Input: part model. Units: mm. Frame: model coordinates. A direction names the side the tool comes from. Round coordinates to 2 decimals unless told otherwise and drop trailing zeros.
Item 1: Mould query, pull axis X, two halves, no side actions, for faces 1 (the flat face through (-12, 50, 13)), 2 (the flat face through (-9, 49, -12.5)), 3 (the cylindrical face through (-14, 18, -13)). Classes: released by +X, released by -X, zero draft, split by the parting line, or undercut.
Item 2: Reachability of faces 4 (the flat face through (6.25, 31, -14)), 5 (the flat face through (14, 31, -6.25)), 6 (the cylindrical face through (-13.732, 49.248, -6.963)) from +Z, -Z, +X, -X, +Y, -Y: full face, straight path, thin tool, end or side. Return the list, or none.
Item 3: Line query: L1, parallel to Y at x = 13.5, z = 8.5; L2, parallel to Z at x = -3.5, y = 47; L3, parallel to Z at x = 3.5, y = 29. Output: solid intervals per line, ascending.
Item 4: First-contact query: pin 1 (2 mm diameter, centred on x = 12, y = 38.5, fed in from +Z); pin 2 (3 mm diameter, centred on y = 44.5, z = 13, fed in from +X); pin 3 (4 mm diameter, centred on x = -4, z = 0, fed in from +Y). Flat tips, straight axial feed; report the tip coordinate or a pass-through.
```python
from build123d import *

# Parameters (mm, degrees)
SKETCH2_W           = 30
SKETCH2_H           = 30
BOSS_EXTRUDE1_DEPTH = 50
SKETCH3_W           = 25
SKETCH3_H           = 25
CUT_EXTRUDE1_DEPTH  = 2.5
FILLET1_R           = 5
SKETCH9_W           = 12.5
SKETCH9_H           = 20.172460503
CUT_EXTRUDE2_DEPTH  = 2.5
CIRPATTERN1_COUNT   = 4
SKETCH10_R          = 21.055389581
CUT_EXTRUDE4_DEPTH  = 5
FILLET2_R           = 2.5


with BuildPart() as part:
    # Sketch2 → Boss-Extrude1 (new body)
    with BuildSketch(Plane(origin=(0, 0, 0), x_dir=(1, 0, 0), z_dir=(0, 1, 0))):
        Rectangle(SKETCH2_W, SKETCH2_H)
    extrude(amount=BOSS_EXTRUDE1_DEPTH)

    # Sketch3 → Cut-Extrude1 (cut)
    with BuildSketch(Plane(origin=(0, 50, 0), x_dir=(1, 0, 0), z_dir=(0, 1, 0))):
        Rectangle(SKETCH3_W, SKETCH3_H)
    extrude(amount=-CUT_EXTRUDE1_DEPTH, mode=Mode.SUBTRACT)

    # Fillet1
    fillet1_edges = [part.edges().sort_by_distance(p)[0] for p in [
        (15, 25, 15),
        (-15, 25, 15),
        (-15, 25, -15),
        (15, 25, -15),
    ]]
    fillet(fillet1_edges, radius=FILLET1_R)

    # Cut-Loft2: read off the stored shape, not the designer's step
    # Cut-Loft2: loft between two sections, ruled curve by curve
    cut_loft2_from = [
        Edge.make_bspline([(0, 0, -12.5), (-25, 0, -12.5), (-25, 0, 12.5), (0, 0, 12.5), (25, 0, 12.5), (25, 0, -12.5), (0, 0, -12.5)], [0, 0, 0, 0, 0.5, 0.5, 0.5, 1, 1, 1, 1], 3, [1, 0.333333333, 0.333333333, 1, 0.333333333, 0.333333333, 1]),
    ]
    cut_loft2_to = [
        Edge.make_bspline([(0.784484005, 47.5, -2.373728048), (-3.962972092, 47.5, -3.942696057), (-5.531940101, 47.5, 0.804760039), (-0.784484005, 47.5, 2.373728048), (3.962972092, 47.5, 3.942696057), (5.531940101, 47.5, -0.804760039), (0.784484005, 47.5, -2.373728048)], [0, 0, 0, 0, 0.5, 0.5, 0.5, 1, 1, 1, 1], 3, [1, 0.333333333, 0.333333333, 1, 0.333333333, 0.333333333, 1]),
    ]
    cut_loft2 = Solid(Shell([*[Face.make_surface_from_curves(cut_loft2_from[k], cut_loft2_to[k]) for k in range(1)], Face(Wire(cut_loft2_from)), Face(Wire(cut_loft2_to))]))
    add(cut_loft2, mode=Mode.SUBTRACT)

    # Sketch9 → Cut-Extrude2 (cut)
    with BuildSketch(Plane.XY.offset(15)):
        with Locations((0, 39.913769749)):
            Rectangle(SKETCH9_W, SKETCH9_H)
    cut_extrude2 = extrude(amount=-CUT_EXTRUDE2_DEPTH, mode=Mode.SUBTRACT)

    # CirPattern1: Cut-Loft2, Cut-Extrude2 ×4 about axis
    cirpattern1_axis = Axis((0, 0, 0), (0, 1, 0))
    add([cut_loft2.rotate(cirpattern1_axis, i * 360 / CIRPATTERN1_COUNT) for i in range(1, CIRPATTERN1_COUNT)], mode=Mode.SUBTRACT)
    add([cut_extrude2.rotate(cirpattern1_axis, i * 360 / CIRPATTERN1_COUNT) for i in range(1, CIRPATTERN1_COUNT)], mode=Mode.SUBTRACT)

    # Sketch10 → Cut-Extrude4 (cut)
    with BuildSketch(Plane(origin=(0, 35, 0), x_dir=(1, 0, 0), z_dir=(0, 1, 0))):
        Circle(SKETCH10_R)
        with BuildLine():
            ThreePointArc((12.5, 10), (11.767766953, 11.767766953), (10, 12.5))
            Line((10, 12.5), (6.25, 12.5))
            Line((6.25, 12.5), (-6.25, 12.5))
            Line((-6.25, 12.5), (-10, 12.5))
            ThreePointArc((-10, 12.5), (-11.767766953, 11.767766953), (-12.5, 10))
            Line((-12.5, 10), (-12.5, 6.25))
            Line((-12.5, 6.25), (-12.5, -6.25))
            Line((-12.5, -6.25), (-12.5, -10))
            ThreePointArc((-12.5, -10), (-11.767766953, -11.767766953), (-10, -12.5))
            Line((-10, -12.5), (-6.25, -12.5))
            Line((-6.25, -12.5), (6.25, -12.5))
            Line((6.25, -12.5), (10, -12.5))
            ThreePointArc((10, -12.5), (11.767766953, -11.767766953), (12.5, -10))
            Line((12.5, -10), (12.5, -6.25))
            Line((12.5, -6.25), (12.5, 6.25))
            Line((12.5, 6.25), (12.5, 10))
        make_face(mode=Mode.SUBTRACT)
    extrude(amount=CUT_EXTRUDE4_DEPTH, mode=Mode.SUBTRACT)

    # Fillet2
    fillet2_edges = [part.edges().sort_by_distance(p)[0] for p in [
        (13.75, 50, -6.25),
        (13.75, 50, 6.25),
        (-6.25, 50, -13.75),
        (6.25, 50, -13.75),
        (-13.75, 50, 6.25),
        (-13.75, 50, -6.25),
        (13.75, 35, 6.25),
        (13.75, 40, 6.25),
        (-6.25, 40, 13.75),
        (-13.75, 40, 6.25),
        (-6.25, 40, -13.75),
        (-13.75, 40, -6.25),
        (6.25, 40, -13.75),
        (13.75, 40, -6.25),
        (6.25, 40, 13.75),
        (-6.25, 35, 13.75),
        (6.25, 35, 13.75),
        (13.75, 35, -6.25),
        (6.25, 35, -13.75),
        (-6.25, 35, -13.75),
        (-13.75, 35, -6.25),
        (-13.75, 35, 6.25),
        (-6.25, 50, 13.75),
    ]]
    fillet(fillet2_edges, radius=FILLET2_R)


solid = part.part
```
From the geometry:
1. face 1: zero draft
1. face 2: undercut
1. face 3: released by -X
2. face 4: -Z, +Y
2. face 5: +X, +Y
2. face 6: +X, -X, +Y
3. L1: y = 0 to 34.99, 40.01 to 49.99
3. L2: z = -12.5 to 12.5
3. L3: z = -15 to -5.28, 5.28 to 15
4. pin 1: stops at z = 12.29
4. pin 2: stops at x = 14.77
4. pin 3: stops at y = 47.5
